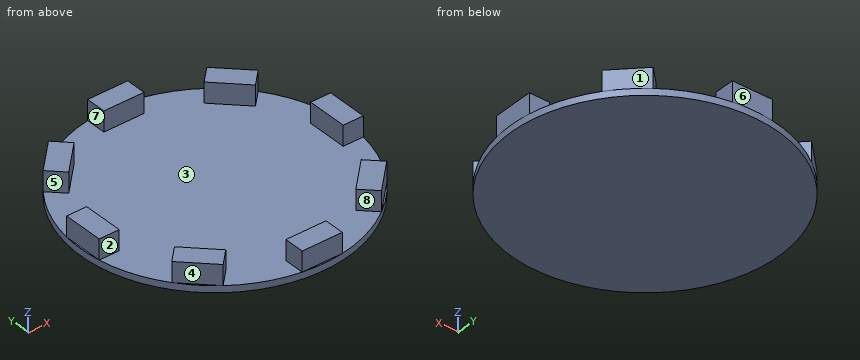
```python
from build123d import *

# Parameters (mm, degrees)
F0_R     = 25.4
F1_DEPTH = 1.27
F2_W     = 3.81
F2_H     = 7.62
F3_DEPTH = 5.08
F4_COUNT = 8


with BuildPart() as f1:
    # F0 (on Top) → F1 (new body)
    with BuildSketch(Plane.XY):
        Circle(F0_R)
    extrude(amount=F1_DEPTH)

    # F2 (on Top) → F3 (join)
    with BuildSketch(Plane.XY):
        with Locations((-23.2076243153, 0)):
            Rectangle(F2_W, F2_H)
    extrude(amount=F3_DEPTH)

    # F4: F1 ×8 about axis
    f4_axis = Axis((0, 0, 1.27), (0, 0, 1))


with BuildPart() as f1_1:
    add(f1.part)
    for i in range(1, F4_COUNT):
        add(f1.part.rotate(f4_axis, i * 360 / F4_COUNT))


solid = f1_1.part
```
Geometry: final body of the model. Coordinates: model frame, mm. Face numbers are marked on the shaded views. A direction names the side the tool comes from. Coordinates: 2 decimals unless noted, no trailing zeros. Loops run counter-clockwise (first coordinate to the right, second up) from the corner with the lowest first, then second, coordinate; pieces in that order, holes last. Notation, with made-up numbers: M -39.5,77.25 L 14.5,77.25 A11 cw 14.5,98.25 Z; hole C 64,43.25 d5. An arc over 180 degrees is marked long. Put each result on its own line as item: value.
(1) Material intervals for probe 1 along X at (y, z) = (0.5, 3.5); probe 2 along Y at (x, z) = (22.5, 3.4); probe 3 along Z at (x, y) = (-5, 19.5), sorted ascending.
Answer sheet:
probe 1: x = -25.11 to -21.3, 21.3 to 25.11
probe 2: y = -3.81 to 3.81
probe 3: z = 0 to 1.27
(2) First-contact query: pin 1 (2 mm diameter, centred on y = -3.5, z = 2, fed in from -X); pin 2 (1.9 mm diameter, centred on y = 23.5, z = 4, fed in from -X); pin 3 (3 mm diameter, centred on y = -1, z = 3.5, fed in from -X); pin 4 (1.6 mm diameter, centred on x = -19, y = -18.5, fed in from +Z). Flat tips, straight axial feed; report the tip coordinate or a pass-through.
Answer sheet:
pin 1: stops at x = -25.24
pin 2: stops at x = -3.81
pin 3: stops at x = -25.11
pin 4: passes through
(3) Cut plane A-A on z = 2.3. State how many separate pieces and enclosed holes the cut face has, then the cut area to 3 significant figures.
Answer sheet:
separate pieces: 8
enclosed holes: 0
area: 232 mm^2
(4) Cut plane D-D on y = -6. Return the cut outline in (x, z).
Answer sheet:
outline: M -24.68,0 L 24.68,0 L 24.68,1.27 L -24.68,1.27 Z
(5) Draft query along X for the marked faces 1, 2 and 3. Return one class per face: pulls with the +X half, pulls with the -X half, needs draft (parallel to the pull), parting line crosses it, or undercut.
Answer sheet:
face 1: pulls with the +X half
face 2: needs draft
face 3: undercut
(6) Cut plane B-B on y = 0. Return the cut outline in (x, z), then the cut area to 3 significant figures.
Answer sheet:
outline: M -25.4,0 L 25.4,0 L 25.4,1.27 L 25.11,1.27 L 25.11,5.08 L 21.3,5.08 L 21.3,1.27 L -21.3,1.27 L -21.3,5.08 L -25.11,5.08 L -25.11,1.27 L -25.4,1.27 Z
area: 93.5 mm^2
(7) Access query for the marked faces 4, 5, 6, 7 and 8. Directions: +Z, -Z, +X, -X, +Y, -Y. A direction counts if a zero-diameter tool reaches every point of the face in a straight line with its end or side. Return the directions, or none.
Answer sheet:
face 4: +Z, -X, -Y
face 5: +Z, -X
face 6: +Z, +X, -X, +Y
face 7: +Z, -X, +Y, -Y
face 8: +Z, -Y
